Autodesk Inventor part; units mm, degrees
ref_plane "YZ Plane" through (0, 0, 0) normal (1, 0, 0) x (0, 1, 0)
ref_plane "XZ Plane" through (0, 0, 0) normal (0, 1, 0) x (-1, 0, 0)
ref_plane "XY Plane" through (0, 0, 0) normal (0, 0, 1) x (1, 0, 0)
sketch "Sketch1" plane through (0, 0, 0) normal (0, 0, 1) x (1, 0, 0)
  line L0 (-27.2578, 3.3251) -> (156.8922, 3.3251)
  line L1 (156.8922, 3.3251) -> (156.8922, -9.3749)
  line L2 (156.8922, -9.3749) -> (-27.2578, -9.3749)
  line L3 (-27.2578, -9.3749) -> (-27.2578, 3.3251)
  line L4 (64.8172, -3.0249) -> (-20.7173, -3.0249)
  line L5 (-20.7173, -3.0249) -> (150.3517, -3.0249)
  line L6 (-20.7173, -3.0249) -> (-20.7173, -5.5649)
  circle A0 centre (-20.7173, -5.5649) radius 1.9812
  circle A1 centre (150.3517, -5.5649) radius 1.9812
  point P0 (0, 0)
  dimension "d0" = 184.15
  dimension "d1" = 12.7
  dimension "d2" = 85.5345
  dimension "d3" = 171.069
  dimension "d4" = 2.54
  dimension "d5" = 3.9624
extrude "Extrusion1" add sketch "Sketch1" along normal blind 3.175
sketch "Sketch2" plane through (-27.2578, 3.3251, 0) normal (0, 1, 0) x (1, 0, 0)
  line L0 (0, -3.175) -> (184.15, -3.175)
  line L1 (184.15, 0) -> (184.15, -3.175)
  line L2 (0, 0) -> (184.15, 0)
  line L3 (0, 0) -> (0, -3.175)
  point P0 (27.2578, 0)
extrude "Extrusion2" add sketch "Sketch2" along normal blind 6.35
sketch "Sketch3" plane through (0, 0, 3.175) normal (0, 0, 1) x (1, 0, 0)
  circle A0 centre (150.3517, -5.5649) radius 1.9812
  circle A1 centre (-20.7173, -5.5649) radius 1.9812
  point P0 (0, 0)
extrude "Extrusion3" add sketch "Sketch3" against normal blind 6.35
sketch "Sketch4" plane through (0, 0, 3.175) normal (0, 0, 1) x (1, 0, 0)
  line L0 (156.8922, -9.3749) -> (-27.2578, -9.3749)
  line L1 (64.8172, -9.3749) -> (64.8172, -5.5649)
  line L2 (64.8172, -5.5649) -> (-17.7328, -5.5649)
  circle A0 centre (-17.7328, -5.5649) radius 1.9812
  line L3 (-17.7328, -5.5649) -> (147.3672, -5.5649)
  circle A1 centre (147.3672, -5.5649) radius 1.9812
  point P0 (0, 0)
  dimension "d12" = 3.81
  dimension "d13" = 82.55
  dimension "d14" = 3.9624
  dimension "d15" = 165.1
extrude "Extrusion4" cut sketch "Sketch4" against normal blind 6.35
sketch "Sketch5" plane through (156.8922, -9.3749, 3.175) normal (1, 0, 0) x (0, 0, -1)
  line L0 (0, 19.05) -> (0, 0)
  line L1 (3.175, 0) -> (0, 0)
  line L2 (3.175, 19.05) -> (3.175, 0)
  line L3 (3.175, 19.05) -> (0, 19.05)
  point P0 (3.175, 9.3749)
extrude "Extrusion5" cut sketch "Sketch5" against normal blind 3.81
sketch "Sketch6" plane through (-27.2578, -9.3749, 0) normal (-1, 0, 0) x (0, 0, 1)
  line L0 (3.175, 0) -> (3.175, 19.05)
  line L1 (3.175, 19.05) -> (0, 19.05)
  line L2 (0, 0) -> (0, 19.05)
  line L3 (0, 0) -> (3.175, 0)
  point P0 (0, 9.3749)
extrude "Extrusion6" cut sketch "Sketch6" against normal blind 2.54
sketch "Sketch7" plane through (0, 0, -3.175) normal (0, 0, -1) x (-1, 0, 0)
  arc A0 (-148.8595, -4.2617) -> (-148.8595, -6.8681) centre (-147.3672, -5.5649) ccw
  arc A1 (-148.8595, -4.2617) -> (-148.8595, -6.8681) centre (-150.3517, -5.5649) ccw
  point P0 (0, 0)
extrude "Extrusion7" cut sketch "Sketch7" against normal blind 3.175
sketch "Sketch8" plane through (0, 0, -3.175) normal (0, 0, -1) x (-1, 0, 0)
  arc A0 (19.225, -6.8681) -> (19.225, -4.2617) centre (17.7328, -5.5649) ccw
  arc A1 (19.225, -6.8681) -> (19.225, -4.2617) centre (20.7173, -5.5649) ccw
  point P0 (0, 0)
extrude "Extrusion8" cut sketch "Sketch8" against normal blind 3.175
sketch "Sketch9" plane through (0, 0, 0) normal (0, 0, -1) x (-1, 0, 0)
  line L0 (-153.0822, -9.3749) -> (24.7178, -9.3749)
  circle A0 centre (-147.3672, -5.5649) radius 1.9812
  line L1 (-147.3672, -5.5649) -> (-102.5362, -5.5649)
  line L2 (-102.5362, -5.5649) -> (-102.5362, -50.3959)
  circle A1 centre (-102.5362, -50.3959) radius 46.0375
  point P0 (0, 0)
  dimension "d26" = 44.831
  dimension "d27" = 44.831
  dimension "d28" = 92.075
extrude "Extrusion9" cut sketch "Sketch9" against normal blind 25.4 contours A1 L1 L2 L0 | L0 A1 | L2 L1 A1 L0
properties part number "small"
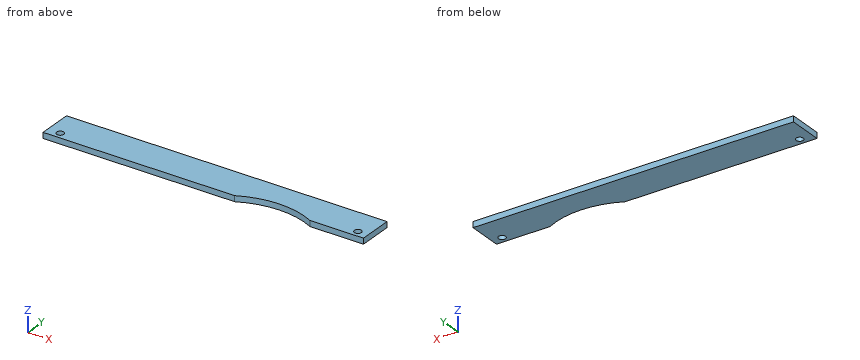
Check sheet for the modelled part. Datum: model origin and axes. Units: mm. Coordinates: 2 decimals unless noted, no trailing zeros. Write each loop counter-clockwise with the first axis right and the second up, starting at its lowest first coordinate (ties: lowest second). Pieces come first, ordered by that corner, then holes. Notation, with made-up numbers: M -26.75,20 L 19.25,20 A26 ccw 19.25,39 Z; hole C 54.5,53.5 d4. An arc over 180 degrees is marked long. Use one line per item in the form item = value.
Item 1: Material ranges on L1, parallel to X at y = -8.5, z = 2.05; L2, parallel to Y at x = 110.5, z = 0.15; L3, parallel to Y at x = 89, z = 1.3, recorded low to high. Write a range as from..to.
Answer below:
L1 = -24.72..83.45, 121.62..153.08
L2 = -5.05..9.68
L3 = -6.39..9.68
Item 2: Sectioned sample at A-A, the plane z = 2.5. Record the cut outline in (x, y) (1 decimal).
Answer below:
outline = M -24.7,-9.4 L 81.6,-9.4 A46 cw 123.4,-9.4 L 153.1,-9.4 L 153.1,9.7 L -24.7,9.7 Z; hole C -17.7,-5.6 d4; hole C 147.4,-5.6 d4
Item 3: Sectioned sample at B-B, the plane x = 112. Record the cut outline in (y, z) (3 decimals).
Answer below:
outline = M -5.342,0 L 9.675,0 L 9.675,3.175 L -5.342,3.175 Z
Item 4: Gauge pin test, flat ends, axial feed: pin 1 Ø3 at (x, y) = (147.37, -5.56) entering from +Z; pin 2 Ø1 at (x, z) = (84, 1.5) entering from -Y. Record the tip position at first contact, or that the pin passes through.
Answer below:
pin_1 = through
pin_2 = -8.48
